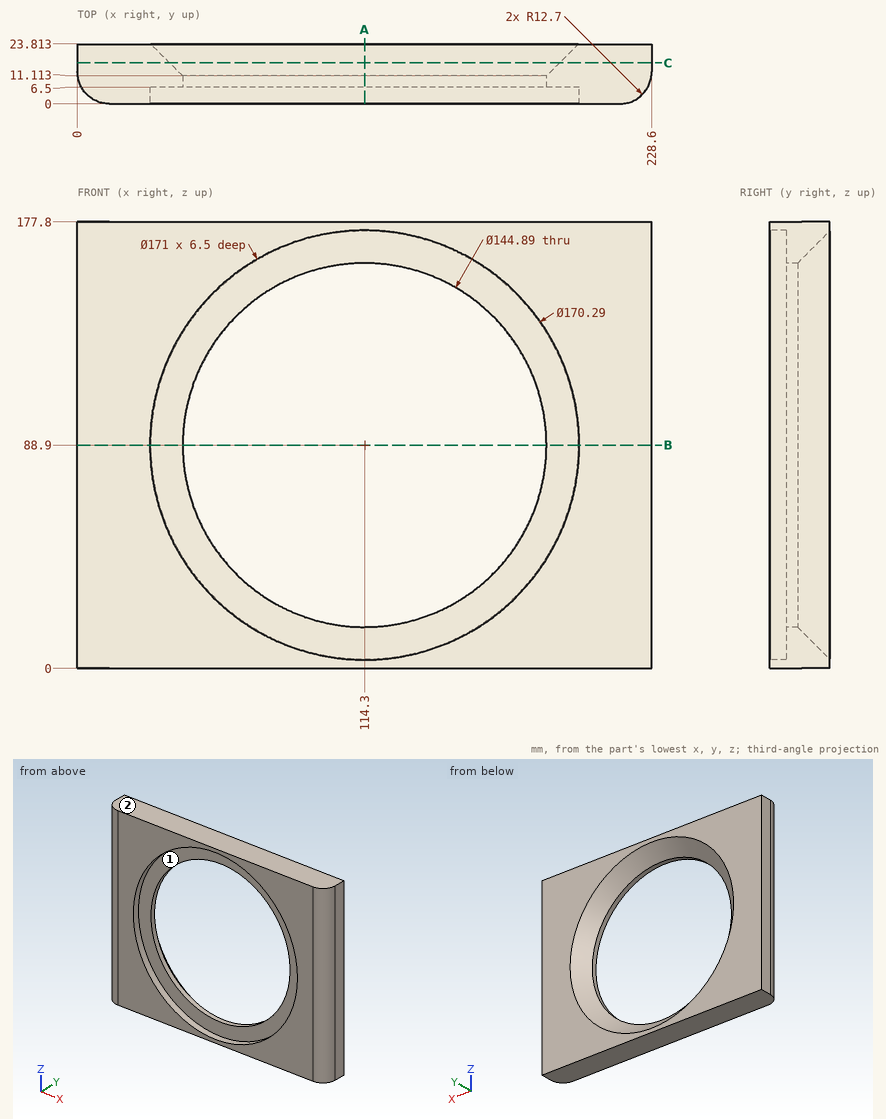
Could you check a few things on this drawing? It's one solid part, dimensions in mm from its lowest x, y, z. A direction names the side the tool comes from. Round coordinates to 2 decimals unless told otherwise and drop trailing zeros. Order: outer loops, then holes, each group sorted by start corner. A loop starts at its lowest first (then second) coordinate and runs counter-clockwise, first axis right, second up.
(1) Imagine slicing it at A-A (x = 114.3). Write out the boundary of the cut face in (y, z) (1 decimal).
Response values:
outline: (0, 0) - (23.8, 0) - (23.8, 3.8) - (11.1, 16.5) - (6.5, 16.5) - (6.5, 3.4) - (0, 3.4) - close; (0, 174.4) - (6.5, 174.4) - (6.5, 161.3) - (11.1, 161.3) - (23.8, 174) - (23.8, 177.8) - (0, 177.8) - close
(2) Which directions (+Z, -Z, +X, -X, +Y, -Y) give clear straight access to the entire face, cutting with the end or side of a thin tool? Please do the marked faces 1 and 2.
Response values:
face 1: -Y
face 2: +Z, +X, -X, +Y, -Y
(3) Please list where these lines run through material, in increasing order: line 1 along Z through (x, y) = (114.3, 1.75); line 2 along Z through (x, y) = (114.3, 8.2) (1 decimal); line 3 along X through (y, z) = (12, 80).
Response values:
line 1: z = 0 to 3.4, 174.4 to 177.8
line 2: z = 0 to 16.5, 161.3 to 177.8
line 3: x = 0.02 to 41.51, 187.09 to 228.58
(4) I'm going to push flat-ended pins straight in: pin 1 (10 mm diameter, centred on y = 6.5, z = 34, fed in from -X); pin 2 (1.5 mm diameter, centred on y = 3, z = 71.5, fed in from +X); pin 3 (8 mm diameter, centred on y = 5, z = 24.5, fed in from -X). Where does each tip first touch, or does it pass through?
Response values:
pin 1: stops at x = 0.06
pin 2: stops at x = 224.91
pin 3: stops at x = 0.55
(5) Imagine slicing it at B-B (z = 88.9). Write out the boundary of the cut face in (x, y) (1 decimal).
Response values:
outline: (0, 12.7) arc R12.7 ccw to (12.7, 0) - (28.8, 0) - (28.8, 6.5) - (41.9, 6.5) - (41.9, 11.1) - (29.2, 23.8) - (0, 23.8) - close; (186.7, 6.5) - (199.8, 6.5) - (199.8, 0) - (215.9, 0) arc R12.7 ccw to (228.6, 12.7) - (228.6, 23.8) - (199.4, 23.8) - (186.7, 11.1) - close
(6) Imagine slicing it at C-C (y = 16.25). Write out the boundary of the cut face in (x, z) (1 decimal), plus the area to 3 significant figures.
Response values:
outline: (0, 0) - (228.6, 0) - (228.6, 177.8) - (0, 177.8) - close; hole circle Ø155.2 at (114.3, 88.9)
area: 21,700 mm2
